Drawing for the job (mm, zero at the part's lowest x, y, z). Round coordinates to 2 decimals unless told otherwise and drop trailing zeros. Write each loop counter-clockwise with the first axis right and the second up, starting at its lowest first coordinate (ties: lowest second). Pieces come first, ordered by that corner, then holes. Notation, with made-up numbers: (62, 35) -> (93, 35) arc R23 ccw to (93, 52) -> close; hole circle Ø8 at (-39, -29). An arc over 180 degrees is marked (long way). Answer in a Markdown table with one row per item. Add a question column.
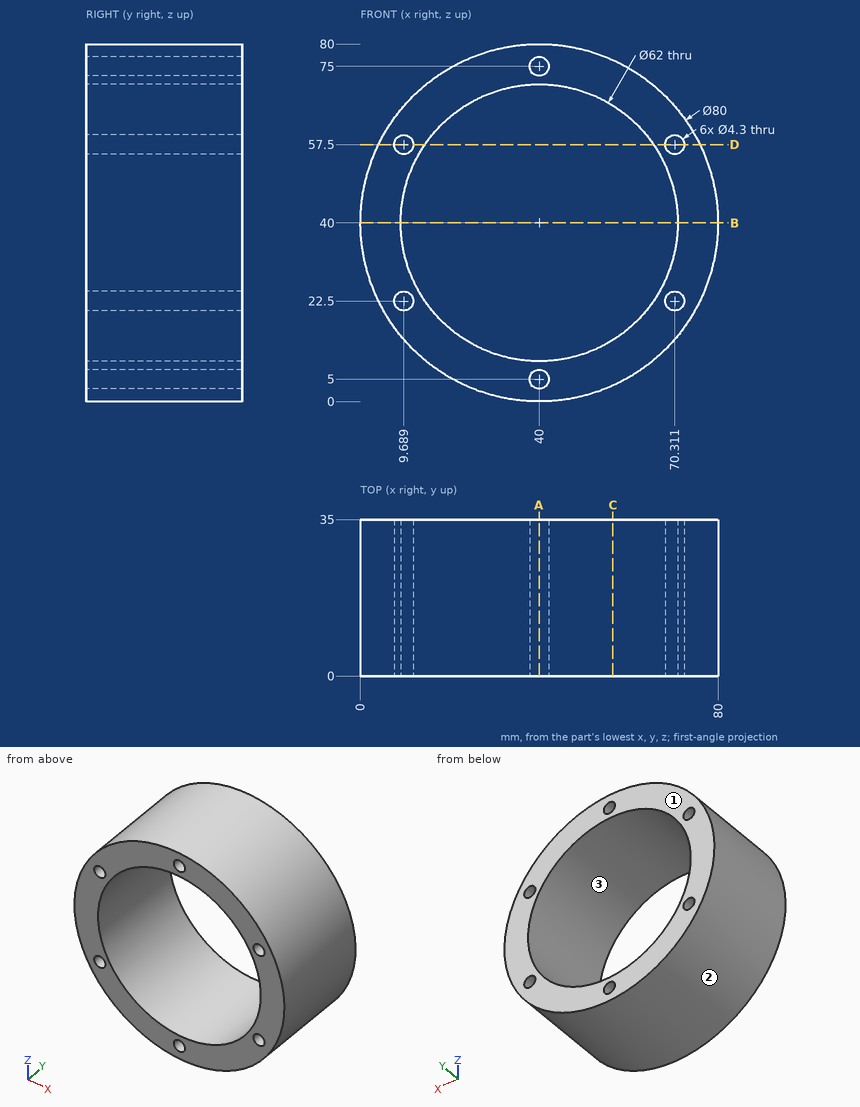
(1) Probe line 1 along X through (y, z) = (18, 22); line 2 along X through (y, z) = (26, 22.5); line 3 along Z through (x, y) = (8, 10.5). List the from-to ranges inside material, lowest first.
(2) Saw through at C-C (x = 56.5). List the corners of the cut face in (y, z).
(3) Saw through at A-A (x = 40). List the corners of the cut face in (y, z).
(4) Saw through at B-B (z = 40). List the corners of the cut face in (x, y), plus the area to 3 significant figures.
(5) Saw through at D-D (z = 57.5). List the corners of the cut face in (x, y), plus the area to 3 significant figures.
(6) Drop flat-ended pins along their axis: P1, Ø2, axis at y = 25, z = 33, coming from the -X side; P2, Ø5, axis at x = 64.5, y = 26.5, coming from the -Z side; P3, Ø4, axis at y = 9.5, z = 61, coming from the +X side. Give the stop position or say it passes through.
(7) Mould opens along X. For the marked faces 1, 2 and 3 say: pulls with the +X half, pulls with the -X half, needs draft (parallel to the pull), parting line crosses it, or undercut.
Answer sheet:
| question | item | result |
|---|---|---|
| 1 | line 1 | x = 4.28 to 7.6, 11.78 to 14.76, 65.24 to 68.22, 72.4 to 75.72 |
| 1 | line 2 | x = 4.03 to 7.54, 11.84 to 14.41, 65.59 to 68.16, 72.46 to 75.97 |
| 1 | line 3 | z = 16 to 21.17, 23.83 to 56.17, 58.83 to 64 |
| 2 | outline | (0, 3.56) -> (35, 3.56) -> (35, 13.76) -> (0, 13.76) -> close; (0, 66.24) -> (35, 66.24) -> (35, 76.44) -> (0, 76.44) -> close |
| 3 | outline | (0, 0) -> (35, 0) -> (35, 2.85) -> (0, 2.85) -> close; (0, 7.15) -> (35, 7.15) -> (35, 9) -> (0, 9) -> close; (0, 71) -> (35, 71) -> (35, 72.85) -> (0, 72.85) -> close; (0, 77.15) -> (35, 77.15) -> (35, 80) -> (0, 80) -> close |
| 4 | outline | (0, 0) -> (9, 0) -> (9, 35) -> (0, 35) -> close; (71, 0) -> (80, 0) -> (80, 35) -> (71, 35) -> close |
| 4 | area | 630 mm² |
| 5 | outline | (4.03, 0) -> (7.54, 0) -> (7.54, 35) -> (4.03, 35) -> close; (11.84, 0) -> (14.41, 0) -> (14.41, 35) -> (11.84, 35) -> close; (65.59, 0) -> (68.16, 0) -> (68.16, 35) -> (65.59, 35) -> close; (72.46, 0) -> (75.97, 0) -> (75.97, 35) -> (72.46, 35) -> close |
| 5 | area | 426 mm² |
| 6 | P1 | stops at x = 0.45 |
| 6 | P2 | stops at z = 6.59 |
| 6 | P3 | stops at x = 75.2 |
| 7 | face 1 | needs draft |
| 7 | face 2 | parting line crosses it |
| 7 | face 3 | undercut |
